Check sheet for the modelled part. Datum: model origin and axes. Units: mm. A direction names the side the tool comes from. Give positions to 0.01 mm unless a question says otherwise; leave off trailing zeros. Order: outer loops, then holes, each group sorted by start corner. A loop starts at its lowest first (then second) coordinate and runs counter-clockwise, first axis right, second up. Notation, with made-up numbers: (70.25, 72) -> (106.25, 72) arc R29 ccw to (106.25, 93) -> close; hole circle Ø6 at (59, 67). An arc over 180 degrees is marked (long way). Answer in a Markdown table with one row per item. Add a question column.
(1) Cross-section at D-D (x = 3.75). Record the cut outline in (y, z), then the cut area to 3 significant figures.
(2) Cross-section at B-B (y = 12.75). Record the cut outline in (x, z), then the cut area to 3 significant figures.
(3) Thickness scan on L1, parallel to Y at x = 3.75, z = -6.9; L2, parallel to X at y = 18.25, z = -8; L3, parallel to Z at x = 16, y = 7.25. Record the ranges inside material, lowest first. Write a range as [from, to].
(4) Cross-section at C-C (y = 3.5). Record the cut outline in (x, z).
(5) Set-up check for faces 5 (the face through (3, 13, -5.7)), 6 (the face through (27, 13, -38.2)), 7 (the face through (0.57, 22.4, -39.47)): record each of +Z, -Z, +X, -X, +Y, -Y from which the full face is reachable in a straight line by a thin tool's end or side.
(6) Cross-section at A-A (y = 7.75). Record the cut outline in (x, z).
(7) Go/stop test with flat-tipped pins: pin 1 (3.5 mm diameter, centred on x = 52, y = 10, fed in from +Z); pin 2 (2 mm diameter, centred on x = 31, y = 5, fed in from +Z); pin 3 (8 mm diameter, centred on x = 37, z = -27, fed in from +Y); pin 4 (3.5 mm diameter, centred on x = 17.25, y = 12.75, fed in from +Z). Record where each tip stops, or that it passes through.
(8) Release check for a two-part mould opening along Y. For faces 1 (the face through (3.49, 19.733, -6.932)), 2 (the face through (50.276, 9.102, -6.932)), 3 (the face through (27, 0, -21)), 4 (the face through (0, 2, -23)) record: released by +Y, released by -Y, zero draft, split by the parting line, or undercut.
```python
from build123d import *

# Parameters (mm, degrees)
SKETCH1_W                   = 55.5
SKETCH1_H                   = 38.2
BRACKETBASE_DEPTH           = 2.5
SKETCH2_W                   = 7
SKETCH2_H                   = 20.5
SERVOMOUNTINGHOLETABS_DEPTH = 2.5
SKETCH3_R                   = 2
SERVOMOUNTINGHOLES_DEPTH    = 2.5
SKETCH4_W                   = 55.5
SKETCH4_H                   = 2.5
BASEWALL_DEPTH              = 23
SKETCH6_R                   = 5.7
BASETRIM_DEPTH              = 2.5
FILLET1_R                   = 2
SKETCH7_R                   = 2
M4MOUNTINGHOLE_DEPTH        = 10


with BuildPart() as part:
    # Sketch1 → bracketBase (new body)
    with BuildSketch(Plane(origin=(0, 0, 0), x_dir=(1, 0, 0), z_dir=(0, 1, 0))):
        with Locations((27.75, 19.1)):
            Rectangle(SKETCH1_W, SKETCH1_H)
    extrude(amount=BRACKETBASE_DEPTH)

    # Sketch2 → servoMountingHoleTabs (add)
    with BuildSketch(Plane.XY.offset(-8.2)):
        with Locations((3.5, 12.75)):
            Rectangle(SKETCH2_W, SKETCH2_H)
        with Locations((52, 12.75)):
            Rectangle(SKETCH2_W, SKETCH2_H)
    extrude(amount=SERVOMOUNTINGHOLETABS_DEPTH)

    # Sketch3 → servoMountingHoles (cut)
    with BuildSketch(Plane.XY.offset(-5.7)):
        with Locations((3.75, 17.75)):
            Circle(SKETCH3_R)
        with Locations(Location((3.75, 7.75, 0), (0, 0, 180))):
            Circle(SKETCH3_R)
        with Locations((51.75, 7.75)):
            Circle(SKETCH3_R)
        with Locations(Location((51.75, 17.75, 0), (0, 0, 180))):
            Circle(SKETCH3_R)
    extrude(amount=-SERVOMOUNTINGHOLES_DEPTH, mode=Mode.SUBTRACT)

    # Sketch4 → baseWall (add)
    with BuildSketch(Plane(origin=(0, 0, 0), x_dir=(1, 0, 0), z_dir=(0, 1, 0))):
        with Locations((27.75, 39.45)):
            Rectangle(SKETCH4_W, SKETCH4_H)
    extrude(amount=BASEWALL_DEPTH)

    # Sketch6 → baseTrim (cut)
    with BuildSketch(Plane(origin=(0, 2.5, 0), x_dir=(1, 0, 0), z_dir=(0, 1, 0))):
        Circle(SKETCH6_R)
        with Locations((55.5, 0)):
            Circle(SKETCH6_R)
    extrude(amount=-BASETRIM_DEPTH, mode=Mode.SUBTRACT)

    # Fillet1
    fillet1_edges = [part.edges().sort_by_distance(p)[0] for p in [
        (0, 23, -6.95),
        (7, 23, -6.95),
        (55.5, 23, -6.95),
        (48.5, 23, -6.95),
        (55.5, 23, -39.45),
        (0, 23, -39.45),
    ]]
    fillet(fillet1_edges, radius=FILLET1_R)

    # Sketch7 → M4mountingHole (cut)
    with BuildSketch(Plane(origin=(0, 0, -40.7), x_dir=(-1, 0, 0), z_dir=(0, 0, -1))):
        with Locations((-17.25, 12.75)):
            Circle(SKETCH7_R)
    extrude(amount=-M4MOUNTINGHOLE_DEPTH, mode=Mode.SUBTRACT)


solid = part.part
```
Answer below:
| question | item | result |
|---|---|---|
| 1 | outline | (0, -40.7) -> (23, -40.7) -> (23, -38.2) -> (2.5, -38.2) -> (2.5, -8.2) -> (5.75, -8.2) -> (5.75, -5.7) -> (2.5, -5.7) -> (2.5, -4.29) -> (0, -4.29) -> close; (9.75, -8.2) -> (15.75, -8.2) -> (15.75, -5.7) -> (9.75, -5.7) -> close; (19.75, -8.2) -> (23, -8.2) -> (23, -5.7) -> (19.75, -5.7) -> close |
| 1 | area | 174 mm² |
| 2 | outline | (0, -40.7) -> (15.25, -40.7) -> (15.25, -38.2) -> (0, -38.2) -> close; (0, -8.2) -> (7, -8.2) -> (7, -5.7) -> (0, -5.7) -> close; (19.25, -40.7) -> (55.5, -40.7) -> (55.5, -38.2) -> (19.25, -38.2) -> close; (48.5, -8.2) -> (55.5, -8.2) -> (55.5, -5.7) -> (48.5, -5.7) -> close |
| 2 | area | 164 mm² |
| 3 | L1 | y = [0, 5.75], [9.75, 15.75], [19.75, 23] |
| 3 | L2 | x = [0, 1.81], [5.69, 7], [48.5, 49.81], [53.69, 55.5] |
| 3 | L3 | z = [-40.7, -38.2] |
| 4 | outline | (0, -40.7) -> (55.5, -40.7) -> (55.5, -38.2) -> (0, -38.2) -> close; (0, -8.2) -> (7, -8.2) -> (7, -5.7) -> (0, -5.7) -> close; (48.5, -8.2) -> (55.5, -8.2) -> (55.5, -5.7) -> (48.5, -5.7) -> close |
| 5 | face 5 | +Z, +X, -X, +Y |
| 5 | face 6 | +X, -X, +Y |
| 5 | face 7 | +Z, -Z, -X, +Y |
| 6 | outline | (0, -40.7) -> (55.5, -40.7) -> (55.5, -38.2) -> (0, -38.2) -> close; (0, -8.2) -> (1.75, -8.2) -> (1.75, -5.7) -> (0, -5.7) -> close; (5.75, -8.2) -> (7, -8.2) -> (7, -5.7) -> (5.75, -5.7) -> close; (48.5, -8.2) -> (49.75, -8.2) -> (49.75, -5.7) -> (48.5, -5.7) -> close; (53.75, -8.2) -> (55.5, -8.2) -> (55.5, -5.7) -> (53.75, -5.7) -> close |
| 7 | pin 1 | stops at z = -5.7 |
| 7 | pin 2 | stops at z = -38.2 |
| 7 | pin 3 | stops at y = 2.5 |
| 7 | pin 4 | passes through |
| 8 | face 1 | undercut |
| 8 | face 2 | undercut |
| 8 | face 3 | released by -Y |
| 8 | face 4 | zero draft |
